Verification items for the finished model (mm, model axes). A direction names the side the tool comes from. Round coordinates to 2 decimals unless told otherwise and drop trailing zeros. Write each loop counter-clockwise with the first axis right and the second up, starting at its lowest first coordinate (ties: lowest second). Pieces come first, ordered by that corner, then holes. Notation, with made-up numbers: M 57,3.25 L 74,3.25 A13 cw 74,13.25 Z; hole C 57,39.5 d1. An arc over 180 degrees is marked long. Write each question's results on one line, items separated by ' | '.
from build123d import *

# Parameters (mm, degrees)
F1_DEPTH = 27
F2_W     = 403.082937
F2_H     = 389.70685
F3_DEPTH = 50


with BuildPart() as f1:
    # F0 (on Top) → F1 (new body)
    with BuildSketch(Plane.XY):
        with BuildLine():
            ThreePointArc((103.141751, 130.827628), (147.000525, 190.646497), (220.000119, 203.797485))
            Line((220.000119, 203.797485), (331.982739, 180.898076))
            ThreePointArc((331.982739, 180.898076), (297.759937, 202.019334), (260.019282, 215.909999))
            ThreePointArc((260.019282, 215.909999), (247.785722, 214.790312), (240.327458, 224.551869))
            ThreePointArc((240.327458, 224.551869), (186.047212, 230.450127), (134.405585, 212.722269))
            ThreePointArc((134.405585, 212.722269), (96.675345, 191.925026), (57.181264, 174.711255))
            ThreePointArc((57.181264, 174.711255), (38.789615, 163.844419), (25.042325, 147.493489))
            ThreePointArc((25.042325, 147.493489), (-75.160431, 14.302014), (-203.064791, -92.567234))
            ThreePointArc((-203.064791, -92.567234), (-248.600788, -164.483519), (-272.445342, -246.19592))
            Line((-272.445342, -246.19592), (-253.424359, -365.238374))
            ThreePointArc((-253.424359, -365.238374), (-248.03197, -364.036727), (-243.660012, -360.659182))
            ThreePointArc((-243.660012, -360.659182), (-226.474264, -324.191868), (-229.146522, -283.966577))
            ThreePointArc((-229.146522, -283.966577), (-222.505303, -205.585554), (-161.231884, -156.257483))
            ThreePointArc((-161.231884, -156.257483), (-11.343038, -29.016538), (103.141751, 130.827628))
        make_face()
    extrude(amount=F1_DEPTH)

    # F2 (on Top) → F3 (cut)
    with BuildSketch(Plane.XY):
        with Locations((-121.900424, -194.853425)):
            Rectangle(F2_W, F2_H)
    extrude(amount=F3_DEPTH, mode=Mode.SUBTRACT)


solid = f1.part
1) Access from +Z, -Z, +X, -X, +Y, -Y to the whole of each face (thin tool, end or side, straight path). Record for faces 4 (the flat face through (-38, 0, 13)), 5 (the flat face through (275.208, 192.508, 13.311)).
Calculated:
face 4: +Z, -Z, +X, -X, -Y | face 5: +Z, -Z, -Y
2) Sectioned sample at D-D, the plane y = 121.5. Record the cut outline in (x, z), and give its area (3 significant figures).
Calculated:
outline: M 9.07,0 L 97.98,0 L 97.98,27 L 9.07,27 Z | area: 2,400 mm²
3) Sectioned sample at A-A, the plane y = 186. Record the cut outline in (x, z).
Calculated:
outline: M 84.17,0 L 140.2,0 L 140.2,27 L 84.17,27 Z; M 307.03,0 L 325.01,0 L 325.01,27 L 307.03,27 Z
4) Material ranges on line 1 (X direction, y = 113, z = 4.5); line 2 (Y direction, x = 54.5, z = 24.5); line 3 (X direction, y = 220, z = 22), recorded low to high. Write a range as [from, to].
Calculated:
line 1: x = [3.51, 93.13] | line 2: y = [52.59, 173.62] | line 3: x = [148.11, 241.93]
5) Sectioned sample at B-B, the plane z = 20. Record the cut outline in (x, y), and give its area (3 significant figures).
Calculated:
outline: M -89.13,0 L 14.12,0 A803.19 ccw 103.14,130.83 A100 cw 220,203.8 L 331.98,180.9 A201.13 ccw 260.02,215.91 A12.7 cw 240.33,224.55 A125.4 ccw 134.41,212.72 A464.72 cw 57.18,174.71 A63.5 ccw 25.04,147.49 A726.99 cw Z | area: 21,400 mm²
6) Draft check along X on faces 1 (the cylindrical face through (61.234, 62.299, 13.311)), 2 (the cylindrical face through (248, 214.7, 13.3)), 3 (the cylindrical face through (39.02, 164.04, 13.31)). Enter one of: pulls with the +X half, pulls with the -X half, needs draft (parallel to the pull), parting line crosses it, or undercut.
Calculated:
face 1: pulls with the +X half | face 2: undercut | face 3: pulls with the -X half
7) Sectioned sample at C-C, the plane x = 171.5. Record the cut outline in (y, z).
Calculated:
outline: M 201.69,0 L 227.95,0 L 227.95,27 L 201.69,27 Z
8) Depth check by flat-ended pin: P1, Ø10, axis at y = 136, z = 15.5, coming from the -X side; P2, Ø3, axis at x = 159.5, z = 24, coming from the -Y side; P3, Ø1, axis at y = 55.5, z = 18, coming from the +X side. Enter the tip coordinate at first touch or a pass-through.
Calculated:
P1: stops at x = 15.08 | P2: stops at y = 196.59 | P3: stops at x = 56.89
